Study the drawing (mm; zero at the part's minimum x, y, z) and answer. A direction names the side the tool comes from. Round coordinates to 2 decimals unless told otherwise and drop trailing zeros. Loops run counter-clockwise (first coordinate to the right, second up) from the corner with the lowest first, then second, coordinate; pieces in that order, holes last. Notation, with made-up numbers: (48, 6) -> (70, 6) arc R20 cw to (70, 37) -> close; hole circle Ø9 at (-3, 89). An arc over 180 degrees is marked (long way). Use one line per item in the form item = value.
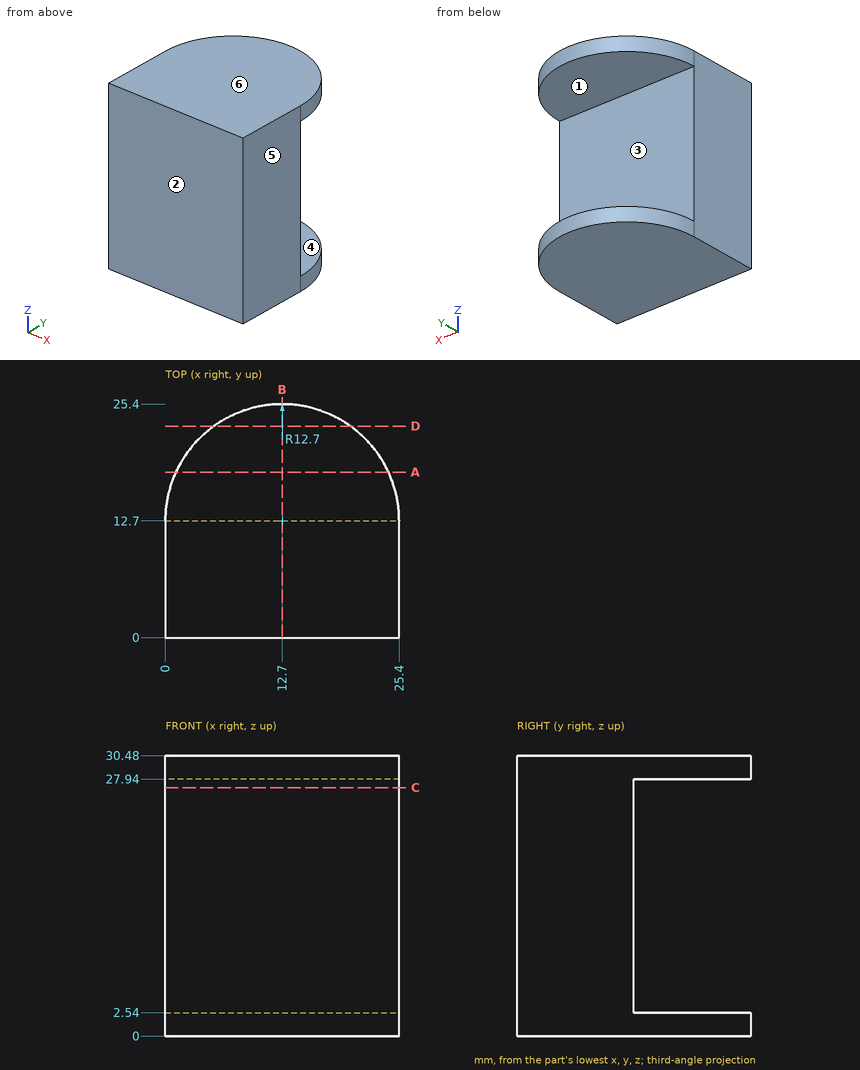
(1) Find section C-C, the plane z = 27. Write down the section's boundary in (x, y).
Completed:
outline = (0, 0) -> (25.4, 0) -> (25.4, 12.7) -> (0, 12.7) -> close
(2) Find section A-A, the plane y = 18. Write down the section's boundary in (x, z).
Completed:
outline = (1.16, 0) -> (24.24, 0) -> (24.24, 2.54) -> (1.16, 2.54) -> close; (1.16, 27.94) -> (24.24, 27.94) -> (24.24, 30.48) -> (1.16, 30.48) -> close
(3) For the marked faces 1 and 2, determine the directions among +Z, -Z, +X, -X, +Y, -Y from which every point of the face is accessible in a straight line to the end or side of a thin tool.
Completed:
face_1 = +X, -X, +Y
face_2 = +Z, -Z, +X, -X, -Y
(4) For a pull along Z with two mould halves and no side action, classify the marked faces 3, 4, 5 and 6 as +Z half, -Z half, draft (parallel to the pull), parting line (faces both ways), or undercut.
Completed:
face_3 = undercut
face_4 = undercut
face_5 = draft
face_6 = +Z half
(5) Find section D-D, the plane y = 23. Write down the section's boundary in (x, z).
Completed:
outline = (5.27, 0) -> (20.13, 0) -> (20.13, 2.54) -> (5.27, 2.54) -> close; (5.27, 27.94) -> (20.13, 27.94) -> (20.13, 30.48) -> (5.27, 30.48) -> close
(6) Consider L1, parallel to Z at x = 9.75, y = 20.25; L2, parallel to Y at x = 14, z = 14. Determine where each line is inside the solid, lowest interval first.
Completed:
L1 = 0 to 2.54, 27.94 to 30.48
L2 = 0 to 12.7
(7) Given P1, Ø1.5, axis at x = 5.5, z = 25.5, coming from the +Y side, flat-ended and moving along its own axis, determine where the tip first touches the part or whether it passes through.
Completed:
P1 = 12.7
(8) Find section B-B, the plane x = 12.7. Write down the section's boundary in (y, z), then the cut area to 3 significant figures.
Completed:
outline = (0, 0) -> (25.4, 0) -> (25.4, 2.54) -> (12.7, 2.54) -> (12.7, 27.94) -> (25.4, 27.94) -> (25.4, 30.48) -> (0, 30.48) -> close
area = 452 mm2
